For this review, take the finished solid that the model builds, in its own axes (mm). A direction names the side the tool comes from. Give positions to 0.01 mm unless a question says otherwise; leave off trailing zeros. Write each loop counter-clockwise with the first axis right and the second up, starting at its lowest first coordinate (ties: lowest second). Pieces come first, ordered by that corner, then holes. Notation, with made-up numbers: M 55,-12 L 80,-12 A11 ccw 80,2 Z; hole C 6,71.5 d2. An arc over 180 degrees is marked long. One line per item, written item: value. Start each with the question number.
Item 1: Consider section C-C, the plane y = 22. Write out the cut boundary in (x, z).
Item 2: To check wall thickness, follow probe 1 along Y at (x, z) = (21.25, 4.25); probe 2 along Y at (x, z) = (4.5, 9); probe 3 along X at (y, z) = (31.5, 9). State the ranges of each line that lie inside material, in increasing order.
Item 3: Tool access review of faces 5 (the face through (8.114, 4.22, 4.93)), 6 (the face through (2, 0, 5)), 7 (the face through (6.9, 4.9, 0)), 8 (the face through (2.792, 28.627, 4.93)): name each direction out of +Z, -Z, +X, -X, +Y, -Y from which nothing blocks a thin tool from reaching the whole face with its end or side.
Item 4: Consider section B-B, the plane z = 6.25. Write out the cut boundary in (x, y), and give its area (3 significant figures).
Item 5: Clearance check with flat-ended pins moving along their axes: pin 1 Ø5 at (x, z) = (9.5, 6) entering from -Y; pin 2 Ø1.5 at (x, z) = (18.5, 6) entering from +Y; pin 3 Ø1.5 at (x, z) = (3, 6.5) entering from -Y; pin 4 Ø2 at (x, y) = (23.5, 14.5) entering from +Z. State where each tip first meets the part, or that it passes through.
Item 6: Consider section D-D, the plane x = 9.75. Write out the cut boundary in (y, z).
Item 7: Mouldability with a two-part tool opening along X and no side actions: class faces 1 (the face through (0, 18, 5)), 2 (the face through (6.9, 4.9, 10)), 3 (the face through (0.35, 32.56, 4.93)), 4 (the face through (27.11, 8.7, 4.93)) as released by +X, released by -X, zero draft, split by the parting line, or undercut.
Item 8: Consider section A-A, the plane x = 22. Write out the cut boundary in (y, z) (3 decimals), and give its area (3 significant figures).
```python
from build123d import *

# Parameters (mm, degrees)
F1_DEPTH = 10


with BuildPart() as f1:
    # F0 (on Top) → F1 (new body)
    with BuildSketch(Plane.XY):
        with BuildLine():
            Line((0, 35), (0, 0))
            Line((0, 0), (5, 0))
            ThreePointArc((5, 0), (27.268138, 9.037983), (19.515337, 31.785493))
            ThreePointArc((19.515337, 31.785493), (18.791109, 31.867286), (18.203721, 31.43581))
            Line((18.203721, 31.43581), (17.935476, 31.011956))
            ThreePointArc((17.935476, 31.011956), (17.81454, 30.218384), (18.316033, 29.591577))
            ThreePointArc((18.316033, 29.591577), (26.210162, 14.267979), (14.479586, 1.637717))
            ThreePointArc((14.479586, 1.637717), (12.394446, 1.637374), (10.490482, 2.487509))
            Line((10.490482, 2.487509), (5.670462, 6.001867))
            ThreePointArc((5.670462, 6.001867), (4.331112, 7.465551), (3.666444, 9.334894))
            Line((3.666444, 9.334894), (1.105092, 27.264357))
            ThreePointArc((1.105092, 27.264357), (2.816973, 28.644292), (4.712199, 29.759137))
            ThreePointArc((4.712199, 29.759137), (5.154266, 30.18947), (5.259664, 30.797335))
            Line((5.259664, 30.797335), (5.185379, 31.317331))
            ThreePointArc((5.185379, 31.317331), (4.66625, 32.058139), (3.761852, 32.077026))
            ThreePointArc((3.761852, 32.077026), (2.175949, 31.2104), (0.687881, 30.184836))
            Line((0.687881, 30.184836), (0, 35))
        make_face()
    extrude(amount=F1_DEPTH)


solid = f1.part
```
Model answer:
1. outline: M 0,0 L 1.86,0 L 1.86,10 L 0,10 Z; M 25.23,0 L 27.9,0 L 27.9,10 L 25.23,10 Z
2. probe 1: y = 1.88 to 5.04, 27.58 to 30.74
2. probe 2: y = 0 to 7.2, 29.65 to 32.13
2. probe 3: x = 0 to 0.5, 2.66 to 5.14, 18.25 to 20.03
3. face 5: +Z, -Z, +Y
3. face 6: +Z, -Z, -X, -Y
3. face 7: -Z, +X, -X, +Y, -Y
3. face 8: +Z, -Z
4. outline: M 0,0 L 5,0 A17.5 ccw 19.52,31.79 A1 ccw 18.2,31.44 L 17.94,31.01 A1 ccw 18.32,29.59 A15 cw 14.48,1.64 A5 cw 10.49,2.49 L 5.67,6 A5 cw 3.67,9.33 L 1.11,27.26 A15 cw 4.71,29.76 A1 ccw 5.26,30.8 L 5.19,31.32 A1 ccw 3.76,32.08 A17.5 ccw 0.69,30.18 L 0,35 Z
4. area: 246 mm2
5. pin 1: stops at y = -1.19
5. pin 2: stops at y = 31.9
5. pin 3: stops at y = 0
5. pin 4: passes through
6. outline: M -1.12,0 L 3.03,0 L 3.03,10 L -1.12,10 Z
7. face 1: released by -X
7. face 2: zero draft
7. face 3: undercut
7. face 4: split by the parting line
8. outline: M 2.422,0 L 5.745,0 L 5.745,10 L 2.422,10 Z; M 26.87,0 L 30.193,0 L 30.193,10 L 26.87,10 Z
8. area: 66.5 mm2
